Here's the drawing with two shaded views (mm, measured from the low corner). I have some questions. A direction names the side the tool comes from. Coordinates: 2 decimals unless noted, no trailing zeros. Write each loop counter-clockwise with the first axis right and the second up, starting at its lowest first coordinate (ties: lowest second). Pieces come first, ordered by that corner, then holes.
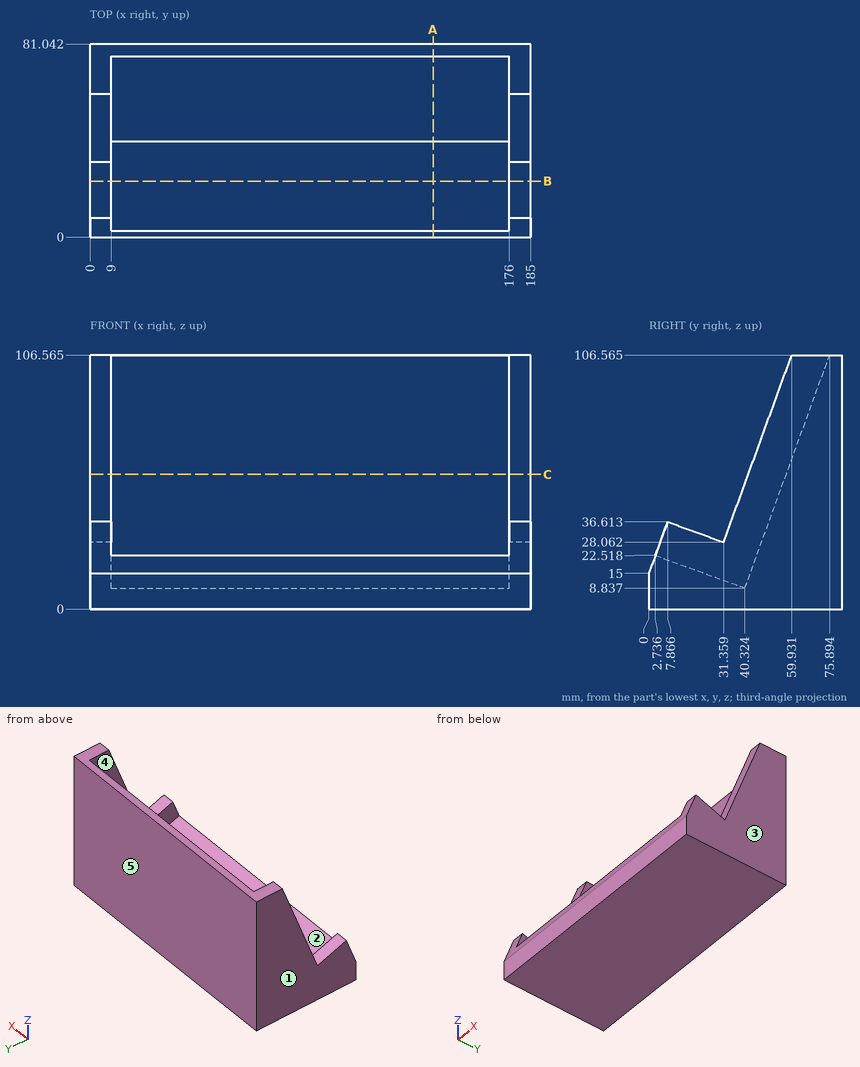
1. Which directions (+Z, -Z, +X, -X, +Y, -Y) give clear straight access to the entire face, cutting with the end or side of a thin tool? Please do the marked faces 1 and 2.
2. If we section it at A-A, the plane x = 144: List the corners of the cut face in (y, z) for me (1 decimal).
3. I'm going to push flat-ended pins straight in: P1, Ø4, axis at x = 75, z = 51.5, coming from the -Y side (1 decimal); P2, Ø10, axis at x = 159, y = 11.5, coming from the +Z side; P3, Ø1, axis at x = 26, z = 90, coming from the -Y side. Where does each tip first touch, or does it pass through?
4. If we section it at C-C, the plane z = 56.5: List the corners of the cut face in (x, y) for me, plus the area to 3 significant figures.
5. If we section it at B-B, the plane y = 23.5: List the corners of the cut face in (x, z) for me.
6. If I drill on L1, parallel to X at y = 21, z = 18.5; L2, parallel to Y at x = 135, z = 78.5; L3, parallel to Y at x = 61, z = 36.5, over which ranges is the centre line in solid material (lowest first)?
7. We'd pull the mould along X, two halves only. Please class the marked faces 3, 4 and 5: released by +X, released by -X, zero draft, split by the parting line, or undercut.
Answers:
1. face 1: +Z, -Z, -X, +Y, -Y
1. face 2: +Z
2. outline: (0, 0) - (81, 0) - (81, 106.6) - (75.9, 106.6) - (40.3, 8.8) - (2.7, 22.5) - (0, 15) - close
3. P1: stops at y = 55.1
3. P2: stops at z = 21.15
3. P3: stops at y = 69.68
4. outline: (0, 41.71) - (9, 41.71) - (9, 57.67) - (176, 57.67) - (176, 41.71) - (185, 41.71) - (185, 81.04) - (0, 81.04) - close
4. area: 4,610 mm2
5. outline: (0, 0) - (185, 0) - (185, 30.92) - (176, 30.92) - (176, 14.96) - (9, 14.96) - (9, 30.92) - (0, 30.92) - close
6. L1: x = 0 to 9, 176 to 185
6. L2: y = 65.68 to 81.04
6. L3: y = 50.39 to 81.04
7. face 3: released by +X
7. face 4: undercut
7. face 5: zero draft
